Model file for the job. Use its own axes, mm. A direction names the side the tool comes from. Round coordinates to 2 decimals unless told otherwise and drop trailing zeros. Order: outer loops, then holes, each group sorted by start corner. A loop starts at its lowest first (then second) coordinate and runs counter-clockwise, first axis right, second up. Notation, with made-up numbers: (77, 42) - (84, 42) arc R25 ccw to (84, 57) - close; hole circle Ø3 at (20.25, -40). An arc over 180 degrees is marked (long way). Use one line per item in the form item = value.
Autodesk Inventor part; units mm, degrees
ref_plane "РабПлоскость1" through (0, 50, 0) normal (0, 1, 0) x (-1, 0, 0)
ref_plane "РабПлоскость2" through (25, 0, 0) normal (1, 0, 0) x (0, 1, 0)
ref_plane "XY Plane" through (0, 0, 0) normal (0, 0, 1) x (1, 0, 0)
sketch "Эскиз1" plane through (0, 0, 0) normal (0, 0, 1) x (1, 0, 0)
  arc A0 (0, -25) -> (0, 25) centre (0, 0) ccw
  arc A1 (0, -20) -> (0, 20) centre (0, 0) ccw
  line L0 (0, 25) -> (0, 20)
  line L1 (0, -25) -> (0, -20)
revolve "Вращение1" add sketch "Эскиз1" angle 360 about axis through (0, -25, 0) along (0, 1, 0)
ref_plane "РабПлоскость1" through (0, 50, 0) normal (0, 1, 0) x (-1, 0, 0)
sketch "Эскиз2" plane through (0, 50, 0) normal (0, 1, 0) x (-1, 0, 0)
  circle A0 centre (0, 0) radius 13
  dimension "d4" = 26
extrude "Выдавливание1" cut sketch "Эскиз2" against normal blind 100
ref_plane "РабПлоскость2" through (25, 0, 0) normal (1, 0, 0) x (0, 1, 0)
sketch "Эскиз3" plane through (25, 0, 0) normal (1, 0, 0) x (0, 1, 0)
  line L0 (-10, 13) -> (-29.0962, 13)
  line L1 (-29.0962, 13) -> (-29.0962, -13)
  line L2 (-29.0962, -13) -> (-10, -13)
  line L3 (-10, -13) -> (-10, 13)
  point P0 (0, 0)
extrude "Выдавливание2" cut sketch "Эскиз3" against normal blind 100
properties part number "шар"
(1) Slice it at D-D on z = 15. Give the cut face in (x, y).
Report:
outline = circle Ø40 at (0, 0); hole circle Ø26.46 at (0, 0)
(2) Pin check, flat tips, straight feed: pin 1 (3.5 mm diameter, centred on x = -15.5, z = -5.5, fed in from -Y); pin 2 (8 mm diameter, centred on x = 10, y = 2, fed in from +Z); pin 3 (1.5 mm diameter, centred on x = -19, y = 12, fed in from -Z); pin 4 (23.5 mm diameter, centred on x = 0, z = 0, fed in from +Y). Stop position of each tip, or through.
Report:
pin_1 = -10
pin_2 = 24.22
pin_3 = -12.38
pin_4 = through
(3) Slice it at B-B on z = -2. Give the cut face in (x, y).
Report:
outline = (-22.83, -10) - (-17.2, -10) arc R19.9 cw to (-12.85, 15.2) - (-12.85, 21.35) arc R24.92 ccw to start; (12.85, 15.2) arc R19.9 cw to (17.2, -10) - (22.83, -10) arc R24.92 ccw to (12.85, 21.35) - close
(4) Slice it at A-A on x = 0. Give the cut face in (y, z).
Report:
outline = (-21.35, -13) arc R25 ccw to (21.35, -13) - (15.2, -13) arc R20 cw to (-15.2, -13) - close; (-21.35, 13) - (-15.2, 13) arc R20 cw to (15.2, 13) - (21.35, 13) arc R25 ccw to start
(5) Probe probe 1 along Z at (x, y) = (8.5, 3.5); probe 2 along Z at (x, y) = (7.5, -7.5); probe 3 along X at (y, z) = (-5.5, -16). List the from-to ranges inside material, lowest first. Write a range as [from, to].
Report:
probe_1 = [-23.25, -17.76], [17.76, 23.25]
probe_2 = [-22.64, -16.96], [16.96, 22.64]
probe_3 = [-18.41, -10.67], [10.67, 18.41]
(6) Tool access for faces 1 (the face through (10.316, 18.32, -7.91)), 2 (the face through (19, -10, 0)): list every direction of +Z, -Z, +X, -X, +Y, -Y with a clear straight run to the whole face (end or side of a thin tool).
Report:
face_1 = +Y, -Y
face_2 = +X, -X, -Y
(7) Slice it at C-C on y = 11.5. Give the cut face in (x, z), then the cut area to 3 significant figures.
Report:
outline = circle Ø44.4 at (0, 0); hole circle Ø32.73 at (0, 0)
area = 707 mm2
